```python
from build123d import *

# Parameters (mm, degrees)
SKETCH1_W            = 508
SKETCH1_H            = 304.8
SKETCH1_W_2          = 431.8
SKETCH1_H_2          = 228.6
BOSS_EXTRUDE1_DEPTH  = 38.1
BOSS_EXTRUDE3_DEPTH  = 19.05
MIRROR3_COPY_1_DEPTH = 19.05


with BuildPart() as part:
    # Sketch1 → Boss-Extrude1 (new body)
    with BuildSketch(Plane(origin=(0, 0, 0), x_dir=(1, 0, 0), z_dir=(0, 1, 0))):
        Rectangle(SKETCH1_W, SKETCH1_H)
        Rectangle(SKETCH1_W_2, SKETCH1_H_2, mode=Mode.SUBTRACT)
    extrude(amount=BOSS_EXTRUDE1_DEPTH)

    # Sketch3 → Boss-Extrude3 (add, symmetric)
    with BuildSketch(Plane(origin=(-50.8, 0, -50.8), x_dir=(0.7071067811865475, 0, -0.7071067811865477), z_dir=(0.7071067811865477, 0, 0.7071067811865475))):
        Polygon((-287.368195874, 38.1), (-398.488889778, -63.5), (-342.026330623, -63.5), (-272.575896933, 0), (-266.942696668, 0), (-266.942696668, 38.1), align=None)
    boss_extrude3 = extrude(amount=BOSS_EXTRUDE3_DEPTH, both=True)

    # Mirror2: Boss-Extrude3 across plane
    add(boss_extrude3.mirror(Plane(origin=(0, 0, 0), x_dir=(0, 0, 1), z_dir=(1, 0, 0))))

    # Mirror3: Boss-Extrude3 across plane
    add(boss_extrude3.mirror(Plane.XY))

    # Mirror3 copy 1 sketch → Mirror3 copy 1 (add, symmetric)
    with BuildSketch(Plane(origin=(50.8, 0, 50.8), x_dir=(-0.7071067811865475, 0, 0.7071067811865477), z_dir=(-0.7071067811865477, 0, -0.7071067811865475))):
        Polygon((-287.368195874, 38.1), (-398.488889778, -63.5), (-342.026330623, -63.5), (-272.575896933, 0), (-266.942696668, 0), (-266.942696668, 38.1), align=None)
    extrude(amount=MIRROR3_COPY_1_DEPTH, both=True)


solid = part.part
```
Input: part model. Units: mm. Frame: model coordinates. A direction names the side the tool comes from. Coordinates: 2 decimals unless noted, no trailing zeros. Write each loop counter-clockwise with the first axis right and the second up, starting at its lowest first coordinate (ties: lowest second). Pieces come first, ordered by that corner, then holes. Notation, with made-up numbers: (9, 56.25) -> (19, 56.25) arc R11 ccw to (19, 60.25) -> close; hole circle Ø9 at (57, -4). An arc over 180 degrees is marked (long way). Answer as a JSON object with one key per item and string values.
1. Section C-C on y = 25. Return the cut outline in (x, z).
Result set:
{"outline": "(-277.6, -149.06) -> (-250.66, -176) -> (-227.06, -152.4) -> (227.06, -152.4) -> (250.66, -176) -> (277.6, -149.06) -> (254, -125.46) -> (254, 125.46) -> (277.6, 149.06) -> (250.66, 176) -> (227.06, 152.4) -> (-227.06, 152.4) -> (-250.66, 176) -> (-277.6, 149.06) -> (-254, 125.46) -> (-254, -125.46) -> close; hole (-215.9, -114.3) -> (215.9, -114.3) -> (215.9, 114.3) -> (-215.9, 114.3) -> close"}
2. Section B-B on z = 103.5. Return the cut outline in (x, y).
Result set:
{"outline": "(-254, 0) -> (-215.9, 0) -> (-215.9, 38.1) -> (-254, 38.1) -> close; (215.9, 0) -> (254, 0) -> (254, 38.1) -> (215.9, 38.1) -> close"}
3. Material intervals for line 1 (Z direction, x = -171, y = 12.5); line 2 (X direction, y = 26, z = 29.5); line 3 (Z direction, x = 295.5, y = -8), sorted ascending. Write a range as from..to.
Result set:
{"line 1": "z = -152.4..-114.3, 114.3..152.4", "line 2": "x = -254..-215.9, 215.9..254", "line 3": "z = -182.2..-166.96, 166.96..182.2"}
4. Mould query, pull axis Z, two halves, no side actions, for faces 5 (the face through (263.5, -11.99, 188.84)), 6 (the face through (-2, 38.1, 120)), 7 (the face through (268.25, -32.195, 167.027)). Classes: released by +Z, released by -Z, zero draft, split by the parting line, or undercut.
Result set:
{"face 5": "released by +Z", "face 6": "zero draft", "face 7": "undercut"}
5. Section D-D on y = -55. Return the cut outline in (x, z).
Result set:
{"outline": "(-339.47, -210.93) -> (-312.53, -237.87) -> (-272.61, -197.95) -> (-299.55, -171.01) -> close; (-339.47, 210.93) -> (-299.55, 171.01) -> (-272.61, 197.95) -> (-312.53, 237.87) -> close; (272.61, -197.95) -> (312.53, -237.87) -> (339.47, -210.93) -> (299.55, -171.01) -> close; (272.61, 197.95) -> (299.55, 171.01) -> (339.47, 210.93) -> (312.53, 237.87) -> close"}
6. First-contact query: P1, Ø19, axis at y = 20.5, z = -32, coming from the -X side; P2, Ø10, axis at y = 23, z = 11, coming from the +X side; P3, Ø4, axis at y = 10.5, z = 125, coming from the -X side; P4, Ø10, axis at x = 139, z = 157, coming from the +Y side. Flat tips, straight axial feed; report the tip coordinate or a pass-through.
Result set:
{"P1": "stops at x = -254", "P2": "stops at x = 254", "P3": "stops at x = -255.54", "P4": "stops at y = 38.1"}
7. Access query for faces 1 (the face through (263.5, -11.99, -188.84)), 2 (the face through (0, 0, -116)), 3 (the face through (-263.5, -11.99, 188.84)), 4 (the face through (-215.9, 19, 2)). Directions: +Z, -Z, +X, -X, +Y, -Y. A direction counts if a zero-diameter tool reaches every point of the face in a straight line with its end or side. Return the directions, or none.
Result set:
{"face 1": "-Z, +Y, -Y", "face 2": "-Y", "face 3": "+Z, +Y, -Y", "face 4": "+Y, -Y"}
8. Section A-A on x = -207.5. Return the cut outline in (y, z), then the cut area to 3 significant figures.
Result set:
{"outline": "(0, -152.4) -> (38.1, -152.4) -> (38.1, -114.3) -> (0, -114.3) -> close; (0, 114.3) -> (38.1, 114.3) -> (38.1, 152.4) -> (0, 152.4) -> close", "area": "2,900 mm2"}
